```python
from build123d import *

# Parameters (mm, degrees)
F0_W     = 19.05
F0_H     = 28.575
F1_DEPTH = 31.75
F2_W     = 19.84375
F2_H     = 19.05
F3_DEPTH = 19.051
F4_W     = 28.575
F4_H     = 4.7625
F5_DEPTH = 38.1
F6_R     = 2.579688
F7_DEPTH = 31.751


with BuildPart() as f1:
    # F0 (on Top) → F1 (new body)
    with BuildSketch(Plane.XY):
        Rectangle(F0_W, F0_H)
    extrude(amount=F1_DEPTH)

    # F2 (on face) → F3 (cut, through all)
    with BuildSketch(Plane.YZ.offset(9.525)):
        with Locations((0, 9.525)):
            Rectangle(F2_W, F2_H)
    extrude(amount=-F3_DEPTH, mode=Mode.SUBTRACT)

    # F4 (on Right) → F5 (join)
    with BuildSketch(Plane.YZ):
        with Locations((0, 21.43125)):
            Rectangle(F4_W, F4_H)
    extrude(amount=F5_DEPTH)

    # F6 (on face) → F7 (cut, through all)
    with BuildSketch(Plane.XY.offset(31.75)):
        Circle(F6_R)
    extrude(amount=-F7_DEPTH, mode=Mode.SUBTRACT)


solid = f1.part
```
The listing builds one solid part. Answer for the finished solid, in the listing's coordinates (mm). A direction names the side the tool comes from. Round coordinates to 2 decimals unless told otherwise and drop trailing zeros. Loops run counter-clockwise (first coordinate to the right, second up) from the corner with the lowest first, then second, coordinate; pieces in that order, holes last. Notation, with made-up numbers: (-24, 20) - (4, 20) arc R23 ccw to (4, 37) - close; hole circle Ø2 at (56, -16.75). An arc over 180 degrees is marked (long way). Return JSON: item names as keys, results as strings. Group by question number.
1. Each of these flat-tipped pins is pushed along its axis until it touches: P1, Ø4, axis at x = 32.5, y = -7, coming from the -Z side; P2, Ø6, axis at x = 16, y = 8, coming from the +Z side; P3, Ø4, axis at y = 5.5, z = 26, coming from the +X side (3 decimals); P4, Ø6, axis at x = 6.5, y = -7, coming from the -Z side. Where does it stop, or does it pass through?
2. The part is cut by section A-A on x = 0. Determine the outline of the cut face in (y, z).
3. The part is cut by section D-D on x = 8. Determine the outline of the cut face in (y, z), then the cut area to 3 significant figures.
4. The part is cut by section B-B on z = 16. Determine the outline of the cut face in (x, y) (1 decimal), then the cut area to 3 significant figures.
5. Consider probe 1 along Y at (x, z) = (0, 28.5); probe 2 along Y at (x, z) = (7.5, 16.5); probe 3 along Z at (x, y) = (32.5, -13). Determine where each line is inside the solid, lowest interval first.
6. The mould has two halves that part along Y. Classify faces 4 (the flat face through (15, 0, 19.05)), 5 (the flat face through (38.1, 0, 21)), 6 (the flat face through (3, 14.288, 16)): pulls with the +Y half, pulls with the -Y half, needs draft (parallel to the pull), parting line crosses it, or undercut.
7. Which of the six approach directions +Z, -Z, +X, -X, +Y, -Y give full straight-line access (tool end or side, diameter ignored) to faces 1 (the flat face through (9.525, 0, 28)), 2 (the flat face through (0, -9.922, 9)), 3 (the flat face through (9.525, -12, 9))?
Resolved:
{
 "1": {"P1": "stops at z = 19.05", "P2": "stops at z = 23.81", "P3": "stops at x = 9.525", "P4": "stops at z = 0"},
 "2": {"outline": "(-14.29, 0) - (-9.92, 0) - (-9.92, 19.05) - (-2.58, 19.05) - (-2.58, 31.75) - (-14.29, 31.75) - close; (2.58, 19.05) - (9.92, 19.05) - (9.92, 0) - (14.29, 0) - (14.29, 31.75) - (2.58, 31.75) - close"},
 "3": {"outline": "(-14.29, 0) - (-9.92, 0) - (-9.92, 19.05) - (9.92, 19.05) - (9.92, 0) - (14.29, 0) - (14.29, 31.75) - (-14.29, 31.75) - close", "area": "529 mm²"},
 "4": {"outline": "(-9.5, -14.3) - (9.5, -14.3) - (9.5, -9.9) - (-9.5, -9.9) - close; (-9.5, 9.9) - (9.5, 9.9) - (9.5, 14.3) - (-9.5, 14.3) - close", "area": "166 mm²"},
 "5": {"probe 1": "y = -14.29 to -2.58, 2.58 to 14.29", "probe 2": "y = -14.29 to -9.92, 9.92 to 14.29", "probe 3": "z = 19.05 to 23.81"},
 "6": {"face 4": "undercut", "face 5": "needs draft", "face 6": "pulls with the +Y half"},
 "7": {"face 1": "+Z, +X, +Y, -Y", "face 2": "-Z, +X, -X", "face 3": "-Z, +X, +Y, -Y"}
}
